Input: part model. Units: mm. Frame: model coordinates. A direction names the side the tool comes from. Round coordinates to 2 decimals unless told otherwise and drop trailing zeros. Order: outer loops, then holes, each group sorted by start corner. A loop starts at its lowest first (then second) coordinate and runs counter-clockwise, first axis right, second up. Notation, with made-up numbers: (-18.75, -22.5) -> (24.25, -22.5) arc R26 ccw to (24.25, 10.5) -> close; hole circle Ø8 at (28, 81). An arc over 180 degrees is marked (long way). Use a Markdown table: item, result.
from build123d import *

# Parameters (mm, degrees)
F0_R     = 7.825273897
F1_DEPTH = 25.4
F3_DEPTH = 25.4
F5_DEPTH = 25.4
F7_DEPTH = 25.4


with BuildPart() as f1:
    # F0 (on Front) → F1 (new body)
    with BuildSketch(Plane.XZ):
        Polygon((0, 25.4), (-25.4, 25.4), (-25.4, 0), (31.75, 0), (31.75, 14.0331494874), (0, 14.0331494874), align=None)
        with Locations((-15.6803522259, 14.0331494874)):
            Circle(F0_R, mode=Mode.SUBTRACT)
    extrude(amount=F1_DEPTH)

    # F2 (on face) → F3 (cut)
    with BuildSketch(Plane.XY.offset(14.0331494874)):
        with BuildLine():
            ThreePointArc((15.1169737006, -13.5398786525), (15.8111405263, -11.8567285769), (16.0478653305, -10.0515075028))
            ThreePointArc((16.0478653305, -10.0515075028), (15.7801184051, -8.1338066206), (14.9973556185, -6.3627765504))
            ThreePointArc((14.9973556185, -6.3627765504), (14.0730886432, -9.9677288292), (15.1169737006, -13.5398786525))
        make_face()
        with BuildLine():
            ThreePointArc((14.9973556185, -6.3627765504), (15.7801184051, -8.1338066206), (16.0478653305, -10.0515075028))
            ThreePointArc((16.0478653305, -10.0515075028), (15.8111405263, -11.8567285769), (15.1169737006, -13.5398786525))
            ThreePointArc((15.1169737006, -13.5398786525), (23.0254188868, -16.6202802265), (28.1442228705, -9.8504777998))
            ThreePointArc((28.1442228705, -9.8504777998), (22.9123385557, -3.0496657427), (14.9973556185, -6.3627765504))
        make_face()
        with BuildLine():
            ThreePointArc((15.1169737006, -13.5398786525), (14.0730886432, -9.9677288292), (14.9973556185, -6.3627765504))
            ThreePointArc((14.9973556185, -6.3627765504), (2.0458192815, -10.1681828387), (15.1169737006, -13.5398786525))
        make_face()
    extrude(amount=-F3_DEPTH, mode=Mode.SUBTRACT)

    # F4 (on face) → F5 (cut)
    with BuildSketch(Plane.XY.offset(14.0331494874)):
        with BuildLine():
            ThreePointArc((26.9380398095, 0), (31.5529389663, -12.816734396), (26.3349507004, -25.4))
            Line((26.3349507004, -25.4), (31.75, -25.4))
            Line((31.75, -25.4), (31.75, 0))
            Line((31.75, 0), (26.9380398095, 0))
        make_face()
    extrude(amount=-F5_DEPTH, mode=Mode.SUBTRACT)

    # F6 (on face) → F7 (cut)
    with BuildSketch(Plane.XZ.offset(25.4)):
        with BuildLine():
            ThreePointArc((-25.4, 16.0824116319), (-11.8835850118, 25.1770035953), (0, 14.0331494874))
            Line((0, 14.0331494874), (0, 25.4))
            Line((0, 25.4), (-25.4, 25.4))
            Line((-25.4, 25.4), (-25.4, 16.0824116319))
        make_face()
    extrude(amount=-F7_DEPTH, mode=Mode.SUBTRACT)


solid = f1.part
1) Cut plane C-C on z = 12. Return loops of the section in (x, y).
Answer key:
| item | result |
|---|---|
| outline | (-25.4, -25.4) -> (-23.24, -25.4) -> (-23.24, 0) -> (-25.4, 0) -> close; (-8.12, -25.4) -> (26.33, -25.4) arc R18.87 ccw to (26.94, 0) -> (-8.12, 0) -> close; hole (15, -6.36) arc R7 ccw (long way) to (15.12, -13.54) arc R7.04 ccw (long way) to start |
2) Draft query along X for faces 1 (the face through (-12.129, -12.878, 25.194)), 2 (the face through (-25.4, -13, 8)), 3 (the face through (2.046, -9.913, 7.115)), 4 (the face through (0, -25.4, 10)). Return one class per face: released by +X, released by -X, zero draft, split by the parting line, or undercut.
Answer key:
| item | result |
|---|---|
| face 1 | split by the parting line |
| face 2 | released by -X |
| face 3 | undercut |
| face 4 | zero draft |
3) Cut plane D-D on z = 20.5. Return loops of the section in (x, y).
Answer key:
| item | result |
|---|---|
| outline | (-22.99, -25.4) -> (-20.09, -25.4) -> (-20.09, 0) -> (-22.99, 0) -> close; (-11.27, -25.4) -> (-2.88, -25.4) -> (-2.88, 0) -> (-11.27, 0) -> close |
4) Cut plane A-A on x = 19.5. Return loops of the section in (y, z).
Answer key:
| item | result |
|---|---|
| outline | (-25.4, 0) -> (-16.7, 0) -> (-16.7, 14.03) -> (-25.4, 14.03) -> close; (-3, 0) -> (0, 0) -> (0, 14.03) -> (-3, 14.03) -> close |
5) Ray query, probe 1 along X at (y, z) = (-3.75, 8.5); probe 2 along X at (y, z) = (-6, 1.5); probe 3 along X at (y, z) = (-14.5, 4.75). Return the intervals inside material, ascending.
Answer key:
| item | result |
|---|---|
| probe 1 | x = -25.4 to -21.21, -10.15 to 5.99, 12.1 to 17.6, 24.61 to 29.47 |
| probe 2 | x = -25.4 to 3.34, 14.76 to 15.22, 27 to 30.45 |
| probe 3 | x = -25.4 to 3.64, 14.45 to 15.83, 26.39 to 31.44 |
6) Contact query for flat-ended pins moving along their axis: P1, Ø6, axis at x = 8, y = -7, coming from the +Z side; P2, Ø12.5, axis at x = 11, y = -13.5, coming from the +Z side; P3, Ø10, axis at y = -22.5, z = 10.5, coming from the +X side. Output: stop coordinate, or through.
Answer key:
| item | result |
|---|---|
| P1 | passes through |
| P2 | stops at z = 14.03 |
| P3 | stops at x = 30.85 |
7) Cut plane B-B on y = -8.25. Return loops of the section in (x, z).
Answer key:
| item | result |
|---|---|
| outline | (-25.4, 0) -> (2.28, 0) -> (2.28, 14.03) -> (0, 14.03) arc R13.07 ccw to (-25.4, 16.08) -> close; (27.96, 0) -> (31.1, 0) -> (31.1, 14.03) -> (27.96, 14.03) -> close; hole circle Ø15.65 at (-15.68, 14.03) |
8) Set-up query: faces 5 (the face through (16, -15, 14.033)), 6 (the face through (0, 0, 10)). Return all of +Z, -Z, +X, -X, +Y, -Y with unobstructed straight access to the full face (end or side cutting, diameter ignored); none if empty.
Answer key:
| item | result |
|---|---|
| face 5 | +Z, +X, +Y, -Y |
| face 6 | +Z, -Z, +X, -X, +Y |
